Input: part model. Units: mm. Frame: model coordinates. Face numbers are marked on the shaded views. A direction names the side the tool comes from. Coordinates: 2 decimals unless noted, no trailing zeros. Write each loop counter-clockwise with the first axis right and the second up, starting at its lowest first coordinate (ties: lowest second). Pieces come first, ordered by that corner, then holes. Notation, with made-up numbers: (-39.75, 24.5) - (-28.75, 24.5) arc R24 ccw to (-28.75, 41.5) - close; hole circle Ø11 at (81, -34). An arc over 180 degrees is marked (long way). Use a Markdown table: item, result. Add a question column.
Q1. Material intervals for probe 1 along X at (y, z) = (-15.5, 17); probe 2 along Z at (x, y) = (-14, -17); probe 3 along Z at (x, y) = (-32.5, -12.75), sorted ascending. Write a range as from..to.
Q2. Mould query, pull axis Z, two halves, no side actions, for the marked faces 4, 5, 6 and 7. Classes: released by +Z, released by -Z, zero draft, split by the parting line, or undercut.
Q3. Pin query (flat end, axial travel): P1, Ø1.9, axis at y = -13, z = 30, coming from the +X side; P2, Ø1.9, axis at x = -8, z = 27.5, coming from the -Y side; P3, Ø2, axis at x = -4.5, z = -3.5, coming from the -Y side. Return the tip coordinate at first contact, or that it passes through.
Q4. Set-up query: the marked faces 1, 2 and 3. Return all of +Z, -Z, +X, -X, +Y, -Y with unobstructed straight access to the full face (end or side cutting, diameter ignored); none if empty.
Q5. Section query D-D (y = -20.5). Return the cut outline in (x, z), then the cut area to 3 significant figures.
Q6. Section query C-C (z = 11). Return the cut outline in (x, y), then the cut area to 3 significant figures.
Q7. Section query B-B (x = -2.5). Return the cut outline in (y, z).
Q8. Section query A-A (y = -12). Return the cut outline in (x, z), then the cut area to 3 significant figures.
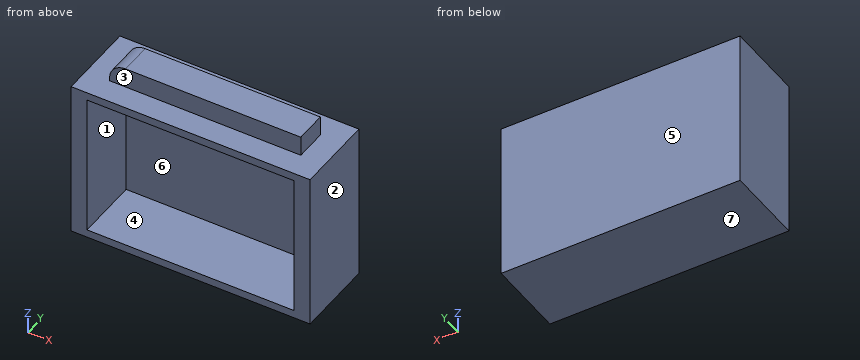
from build123d import *

# Parameters (mm, degrees)
F0_W          = 76.2
F0_H          = 50.8
F1_DEPTH      = 25.4
F2_W          = 66.04
F2_H          = 45.72
F3_DEPTH      = 20.32
F3_DEPTH_BACK = 25.4
F4_W          = 60.9600003704
F4_H          = 10.1600003704
F5_DEPTH      = 6.35
F6_R          = 5.08


with BuildPart() as f1:
    # F0 (on Front) → F1 (new body)
    with BuildSketch(Plane.XZ):
        Rectangle(F0_W, F0_H)
    extrude(amount=F1_DEPTH)

    # F2 (on face) → F3 (cut, two sides)
    with BuildSketch(Plane.XZ.offset(25.4)) as f3_sk:
        Rectangle(F2_W, F2_H)
    extrude(amount=-F3_DEPTH, mode=Mode.SUBTRACT)
    extrude(f3_sk.sketch, amount=F3_DEPTH_BACK, mode=Mode.SUBTRACT)

    # F4 (on face) → F5 (join)
    with BuildSketch(Plane.XY.offset(25.4)):
        with Locations((0, -12.7)):
            Rectangle(F4_W, F4_H)
    extrude(amount=F5_DEPTH)

    # F6
    f6_edges = [f1.edges().sort_by_distance(p)[0] for p in [
        (-30.48, -12.7, 31.75),
    ]]
    fillet(f6_edges, radius=F6_R)


solid = f1.part
Values follow:
| question | item | result |
|---|---|---|
| 1 | probe 1 | -38.1..-33.02, 33.02..38.1 |
| 1 | probe 2 | -25.4..-22.86, 22.86..31.75 |
| 1 | probe 3 | -25.4..-22.86, 22.86..25.4 |
| 2 | face 4 | undercut |
| 2 | face 5 | zero draft |
| 2 | face 6 | undercut |
| 2 | face 7 | released by -Z |
| 3 | P1 | x = 30.48 |
| 3 | P2 | y = -17.78 |
| 3 | P3 | y = -5.08 |
| 4 | face 1 | -Y |
| 4 | face 2 | +Z, -Z, +X, +Y, -Y |
| 4 | face 3 | +Z, +X, -X, -Y |
| 5 | outline | (-38.1, -25.4) - (38.1, -25.4) - (38.1, 25.4) - (-38.1, 25.4) - close; hole (-33.02, -22.86) - (33.02, -22.86) - (33.02, 22.86) - (-33.02, 22.86) - close |
| 5 | area | 852 mm2 |
| 6 | outline | (-38.1, -25.4) - (-33.02, -25.4) - (-33.02, -5.08) - (33.02, -5.08) - (33.02, -25.4) - (38.1, -25.4) - (38.1, 0) - (-38.1, 0) - close |
| 6 | area | 594 mm2 |
| 7 | outline | (-25.4, -25.4) - (0, -25.4) - (0, 25.4) - (-7.62, 25.4) - (-7.62, 31.75) - (-17.78, 31.75) - (-17.78, 25.4) - (-25.4, 25.4) - (-25.4, 22.86) - (-5.08, 22.86) - (-5.08, -22.86) - (-25.4, -22.86) - close |
| 8 | outline | (-38.1, -25.4) - (38.1, -25.4) - (38.1, 25.4) - (30.48, 25.4) - (30.48, 31.75) - (-25.4, 31.75) arc R5.08 ccw to (-30.48, 26.67) - (-30.48, 25.4) - (-38.1, 25.4) - close; hole (-33.02, -22.86) - (33.02, -22.86) - (33.02, 22.86) - (-33.02, 22.86) - close |
| 8 | area | 1,230 mm2 |
